Build history of the part. All positions in model axes, mm. A direction names the side the tool comes from. Give positions to 0.01 mm unless a question says otherwise; leave off trailing zeros. Loops run counter-clockwise (first coordinate to the right, second up) from the corner with the lowest first, then second, coordinate; pieces in that order, holes last. Notation, with made-up numbers: (45.25, 67.25) - (56.25, 67.25) arc R26 cw to (56.25, 97.25) - close; hole circle Ø4 at (-26, 80.25). An arc over 180 degrees is marked (long way). Return JSON: item names as keys, results as strings. Group by question number.
1) Slice it at A-A (y = 6.75). List the corners of the cut face in (x, z), and give its area (3 significant figures).
2) Drill centre lines: probe 1 along X at (y, z) = (5.25, 1.5); probe 2 along Y at (x, z) = (-11.5, -29.5); probe 3 along Z at (x, y) = (6.5, -7.25). Where is each one in solid material? Low to high. Write a range as from..to.
3) Drop flat-ended pins along their axis: pin 1 (10 mm diameter, centred on x = -8, z = -14.5, fed in from +Y); pin 2 (2.5 mm diameter, centred on y = -11, z = 15, fed in from +X); pin 3 (3.5 mm diameter, centred on x = 0, z = 15.5, fed in from +Y). Give the stop position or say it passes through.
4) Mould opens along Y. For faces 6 (the face through (0.049, -13.275, 5.719)), 7 (the face through (0, 12, 3)), 8 (the face through (3, -13, -27)) say: released by +Y, released by -Y, zero draft, split by the parting line, or undercut.
5) Slice it at B-B (x = 10). List the corners of the cut face in (y, z), and give its area (3 significant figures).
6) 3-axis set-ups, long thin cutter, end or side, ignore diameter. For faces 1 (the face through (0, -11, 11)), 2 (the face through (0, -13, 14)), 3 (the face through (22.25, 0, 2)), 4 (the face through (0, -13, -9)), 5 (the face through (1.5, 12, 14)): which of +Z, -Z, +X, -X, +Y, -Y reach the whole face in a straight line?
Autodesk Inventor part; units mm, degrees
ref_plane "YZ Plane" through (0, 0, 0) normal (1, 0, 0) x (0, 1, 0)
ref_plane "XZ Plane" through (0, 0, 0) normal (0, 1, 0) x (-1, 0, 0)
ref_plane "XY Plane" through (0, 0, 0) normal (0, 0, 1) x (1, 0, 0)
sketch "Sketch2" plane through (0, 0, 0) normal (0, 0, 1) x (1, 0, 0)
  line L0 (22.25, 12) -> (-22.25, 12)
  line L1 (-22.25, 12) -> (-22.25, -12)
  line L2 (-22.25, -12) -> (22.25, -12)
  line L3 (22.25, -12) -> (22.25, 12)
  line L4 (22.25, 12) -> (-22.25, -12) construction
  line L5 (-22.25, 12) -> (22.25, -12) construction
  line L6 (24.25, 14) -> (-24.25, 14)
  line L7 (-24.25, 14) -> (-24.25, -14)
  line L8 (-24.25, -14) -> (24.25, -14)
  line L9 (24.25, -14) -> (24.25, 14)
  line L10 (24.25, 14) -> (-24.25, -14) construction
  line L11 (-24.25, 14) -> (24.25, -14) construction
  point P0 (0, 0)
  dimension "d0" = 44.5
  dimension "d1" = 24
  dimension "d2" = 48.5
  dimension "d3" = 28
extrude "Extrusion1" add sketch "Sketch2" along normal blind 5
sketch "Sketch3" plane through (0, 0, 5) normal (0, 0, 1) x (1, 0, 0)
  line L0 (-24.25, 14) -> (-24.25, -14) construction
  line L1 (-24.25, -14) -> (24.25, -14) construction
  line L2 (24.25, -14) -> (24.25, 14) construction
  line L3 (24.25, 14) -> (-24.25, 14) construction
  line L4 (22.25, 12) -> (22.25, -12) construction
  line L5 (22.25, -12) -> (-22.25, -12) construction
  line L6 (-22.25, -12) -> (-22.25, 12) construction
  line L7 (-22.25, 12) -> (22.25, 12) construction
  line L8 (1.5, -13) -> (-1.5, -13)
  line L9 (-1.5, -13) -> (-1.5, -12)
  line L10 (-1.5, -12) -> (1.5, -12)
  line L11 (1.5, -12) -> (1.5, -13)
  line L12 (1.5, -13) -> (-1.5, -12) construction
  line L13 (-1.5, -13) -> (1.5, -12) construction
  line L14 (1.5, 13) -> (-1.5, 13)
  line L15 (-1.5, 13) -> (-1.5, 12)
  line L16 (-1.5, 12) -> (1.5, 12)
  line L17 (1.5, 12) -> (1.5, 13)
  line L18 (1.5, 13) -> (-1.5, 12) construction
  line L19 (-1.5, 13) -> (1.5, 12) construction
  line L20 (0, 19.6) -> (0, -19.6) construction
  point P0 (0, 0)
  point P1 (0, -12.5)
  point P2 (0, -12.5)
  point P3 (0, 12.5)
  point P4 (0, 12.5)
  dimension "d8" = 3
  dimension "d19" = 1
  dimension "d22" = 3
  dimension "d23" = 1
extrude "Extrusion2" add sketch "Sketch3" along normal blind 16.5
sketch "Sketch4" plane through (-22.25, -12, 0) normal (0, 1, 0) x (1, 0, 0)
  line L0 (44.5, 0) -> (0, 0) construction
  line L1 (0, 0) -> (0, -5) construction
  line L2 (20.75, -5) -> (0, -5) construction
  line L3 (20.75, -5) -> (20.75, -21.5) construction
  line L4 (23.75, -21.5) -> (20.75, -21.5) construction
  line L5 (23.75, -5) -> (23.75, -21.5) construction
  line L6 (44.5, -5) -> (23.75, -5) construction
  line L7 (44.5, 0) -> (44.5, -5) construction
  line L8 (20.75, -19) -> (23.75, -19)
  line L9 (23.75, -19) -> (23.75, -10)
  line L10 (23.75, -10) -> (20.75, -10)
  line L11 (20.75, -10) -> (20.75, -19)
  line L12 (20.75, -19) -> (23.75, -10) construction
  line L13 (23.75, -19) -> (20.75, -10) construction
  line L14 (22.25, 4.3) -> (22.25, -25.8) construction
  point P0 (22.25, 0)
  point P1 (22.25, -14.5)
  point P2 (22.25, -14.5)
  dimension "d12" = 10
  dimension "d13" = 9
extrude "Extrusion3" add sketch "Sketch4" along normal blind 2
sketch "Sketch5" plane through (1.5, -14, 5) normal (1, 0, 0) x (0, 0, -1)
  line L0 (0, 2) -> (0, 1) construction
  line L1 (0, 2) -> (-5, 2) construction
  line L2 (-5, 2) -> (-5, 4) construction
  line L3 (-14, 4) -> (-5, 4) construction
  line L4 (-14, 2) -> (-14, 4) construction
  line L5 (-14, 2) -> (-16.5, 2) construction
  line L6 (-16.5, 1) -> (-16.5, 2) construction
  line L7 (0, 1) -> (-16.5, 1) construction
  line L8 (-5, 2) -> (-7, 4)
  line L9 (-5, 2) -> (-5, 4)
  line L10 (-7, 4) -> (-5, 4)
  point P0 (5, 14)
  dimension "d16" = 2
extrude "Extrusion4" cut sketch "Sketch5" against normal up to surface (3 mm away)
sketch "Sketch6" plane through (-22.25, 12, 0) normal (0, -1, 0) x (1, 0, 0)
  line L0 (23.75, 12) -> (20.75, 12) construction
  line L1 (20.75, 10) -> (23.75, 10) construction
  line L2 (23.75, 19) -> (20.75, 19) construction
  line L3 (20.75, 19) -> (23.75, 19)
  line L4 (23.75, 19) -> (23.75, 10)
  line L5 (23.75, 10) -> (20.75, 10)
  line L6 (20.75, 10) -> (20.75, 19)
  point P0 (22.25, 0)
extrude "Extrusion5" add sketch "Sketch6" along normal blind 2
sketch "Sketch8" plane through (1.5, 12, 5) normal (1, 0, 0) x (0, 0, -1)
  line L0 (0, 1) -> (0, 0) construction
  line L1 (0, 1) -> (-16.5, 1) construction
  line L2 (-16.5, 0) -> (-16.5, 1) construction
  line L3 (-14, 0) -> (-16.5, 0) construction
  line L4 (-14, 0) -> (-14, -2) construction
  line L5 (-5, -2) -> (-14, -2) construction
  line L6 (-5, 0) -> (-5, -2) construction
  line L7 (0, 0) -> (-5, 0) construction
  line L8 (-7, -2) -> (-5, 0)
  line L9 (-7, -2) -> (-5, -2)
  line L10 (-5, -2) -> (-5, 0)
  point P0 (5, -12)
  dimension "d26" = 2
extrude "Extrusion6" cut sketch "Sketch8" against normal up to surface (3 mm away)
fillet "Fillet1" radius 2 6 edges at (1.5, -12.5, 5) (0, -13, 5) (-1.5, -12.5, 5) (1.5, 12.5, 5) (0, 13, 5) (-1.5, 12.5, 5)
fillet "Fillet2" radius 1 4 edges at (0, -12, 10) (0, -10, 12) (0, 12, 10) (0, 10, 12)
sketch "Sketch9" plane through (0, 0, 0) normal (0, 0, -1) x (-1, 0, 0)
  line L0 (24.25, 14) -> (24.25, -14) construction
  line L1 (-24.25, 14) -> (24.25, 14) construction
  line L2 (-24.25, -14) -> (-24.25, 14) construction
  line L3 (24.25, -14) -> (-24.25, -14) construction
  line L4 (-22.25, 12) -> (-22.25, -12) construction
  line L5 (22.25, 12) -> (-22.25, 12) construction
  line L6 (22.25, -12) -> (22.25, 12) construction
  line L7 (-22.25, -12) -> (22.25, -12) construction
  line L8 (-24.25, 14) -> (24.25, 14)
  line L9 (24.25, 14) -> (24.25, -14)
  line L10 (24.25, -14) -> (-24.25, -14)
  line L11 (-24.25, -14) -> (-24.25, 14)
  point P0 (0, 0)
extrude "Extrusion7" add sketch "Sketch9" along normal blind 2
fillet "Fillet3" radius 1 2 edges at (0, -12, 19) (0, 12, 19)
fillet "Fillet4" radius 1 2 edges at (0, -10, 19) (0, 10, 19)
sketch "Sketch10" plane through (0, 0, -2) normal (0, 0, -1) x (-1, 0, 0)
  line L0 (-22.25, -12) -> (22.25, -12) construction
  line L1 (-24.25, -14) -> (24.25, -14) construction
  line L2 (24.25, -14) -> (24.25, 14) construction
  line L3 (24.25, 14) -> (-24.25, 14) construction
  line L4 (-24.25, 14) -> (-24.25, -14) construction
  line L5 (-24.25, -14) -> (24.25, -14)
  line L6 (24.25, -14) -> (24.25, -11)
  line L7 (24.25, -11) -> (-24.25, -11)
  line L8 (-24.25, -11) -> (-24.25, -14)
  point P0 (0, 0)
  dimension "d35" = 3
extrude "Extrusion8" add sketch "Sketch10" along normal blind 50
sketch "Sketch11" plane through (3.5, -14, 5) normal (0, -1, 0) x (1, 0, 0)
  line L0 (20.75, -7) -> (-27.75, -7) construction
  line L1 (-3.5, -47) -> (-3.5, -17) construction
  line L2 (-0.5, -47) -> (-0.5, -17)
  line L3 (-6.5, -17) -> (-6.5, -47)
  arc A0 (-6.5, -47) -> (-0.5, -47) centre (-3.5, -47) ccw
  arc A1 (-0.5, -17) -> (-6.5, -17) centre (-3.5, -17) ccw
  line L4 (20.75, -57) -> (-27.75, -57) construction
  line L5 (-3.5, 31.2) -> (-3.5, -71.7) construction
  point P0 (-3.5, -5)
  point P1 (-3.5, -32)
  dimension "d38" = 6
  dimension "d39" = 25
  dimension "d40" = 25
  dimension "d41" = 30
  dimension "d42" = 3
extrude "Extrusion9" cut sketch "Sketch11" against normal blind 10
fillet "Fillet5" radius 2 1 edges at (0, -11, -2)
properties part number "P036_SupportLidar"
Results:
{
 "1": {"outline": "(-24.25, -2) - (24.25, -2) - (24.25, 5) - (22.25, 5) - (22.25, 0) - (-22.25, 0) - (-22.25, 5) - (-24.25, 5) - close", "area": "117 mm2"},
 "2": {"probe 1": "-24.25..-22.25, 22.25..24.25", "probe 2": "-14..-11", "probe 3": "-2..0"},
 "3": {"pin 1": "y = -11", "pin 2": "x = 1.5", "pin 3": "y = 13"},
 "4": {"face 6": "released by -Y", "face 7": "undercut", "face 8": "zero draft"},
 "5": {"outline": "(-14, -52) - (-11, -52) - (-11, -4) arc R2 cw to (-9, -2) - (14, -2) - (14, 5) - (12, 5) - (12, 0) - (-12, 0) - (-12, 5) - (-14, 5) - close", "area": "227 mm2"},
 "6": {"face 1": "+X, -X", "face 2": "+Z, +X, -X, -Y", "face 3": "+Z", "face 4": "+Y, -Y", "face 5": "+Z, +X, +Y, -Y"}
}
